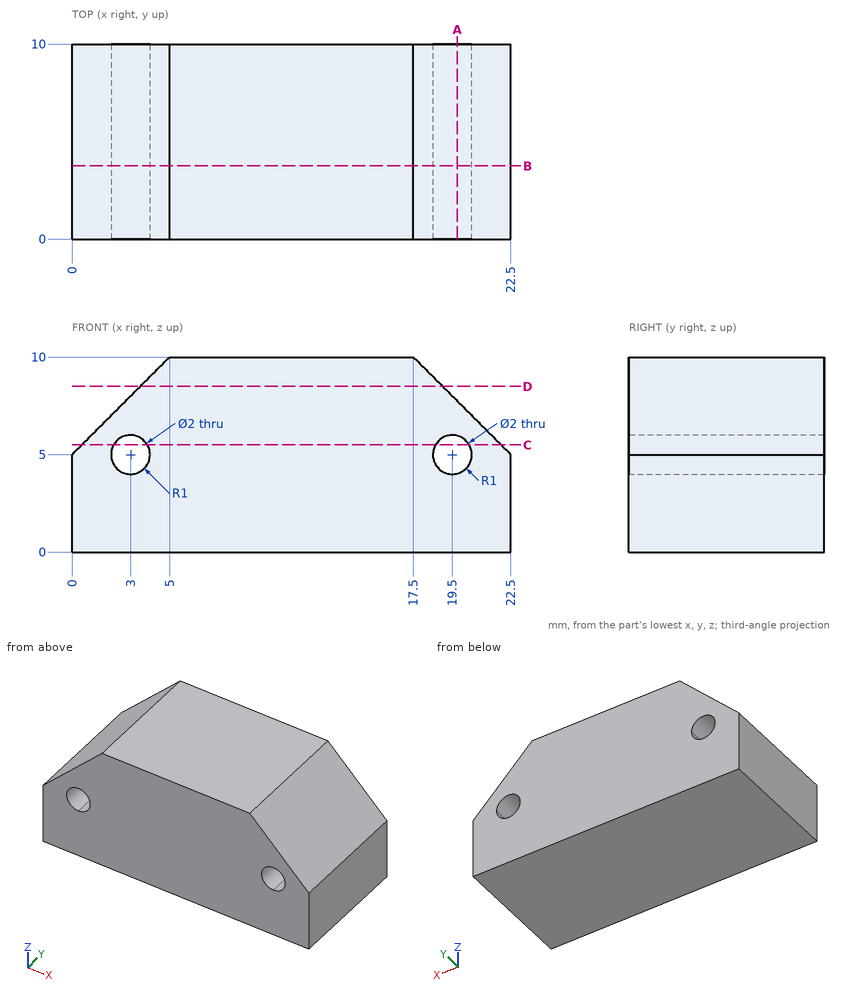
For this review, use the dimensioned drawing (mm, ordinates from the lowest corner) and the shaded views. Give positions to 0.01 mm unless a question says otherwise; leave off trailing zeros. Order: outer loops, then holes, each group sorted by start corner. A loop starts at its lowest first (then second) coordinate and runs counter-clockwise, first axis right, second up. Notation, with made-up numbers: (51.25, 3.25) -> (72.25, 3.25) arc R29 ccw to (72.25, 36.25) -> close; hole circle Ø5 at (-2.5, -4). An arc over 180 degrees is marked (long way). Write item = value, one per line. Start each with the question number.
(1) Take a section at B-B (y = 3.75). Write out the cut boundary in (x, z), plus the area to 3 significant figures.
(2) For pin 1 Ø1 at (y, z) = (4.5, 8) entering from -X, flat-tipped, find the tip position at first contact; note if it passes through.
(3) Take a section at C-C (z = 5.5). Write out the cut boundary in (x, y), plus the area to 3 significant figures.
(4) Take a section at D-D (z = 8.5). Write out the cut boundary in (x, y), plus the area to 3 significant figures.
(5) Take a section at A-A (x = 19.75). Write out the cut boundary in (y, z).
(6) For L1, parallel to X at y = 2.25, z = 5.25; L2, parallel to X at y = 8, z = 7; L3, parallel to Z at x = 3, y = 7, list the stretches that pass through material, from the lowest coordinate up. Write a range as from..to.
Returned:
q1.outline = (0, 0) -> (22.5, 0) -> (22.5, 5) -> (17.5, 10) -> (5, 10) -> (0, 5) -> close; hole circle Ø2 at (3, 5); hole circle Ø2 at (19.5, 5)
q1.area = 194 mm²
q2.pin_1 = 2.5
q3.outline = (0.5, 0) -> (2.13, 0) -> (2.13, 10) -> (0.5, 10) -> close; (3.87, 0) -> (18.63, 0) -> (18.63, 10) -> (3.87, 10) -> close; (20.37, 0) -> (22, 0) -> (22, 10) -> (20.37, 10) -> close
q3.area = 180 mm²
q4.outline = (3.5, 0) -> (19, 0) -> (19, 10) -> (3.5, 10) -> close
q4.area = 155 mm²
q5.outline = (0, 0) -> (10, 0) -> (10, 4.03) -> (0, 4.03) -> close; (0, 5.97) -> (10, 5.97) -> (10, 7.75) -> (0, 7.75) -> close
q6.L1 = 0.25..2.03, 3.97..18.53, 20.47..22.25
q6.L2 = 2..20.5
q6.L3 = 0..4, 6..8
